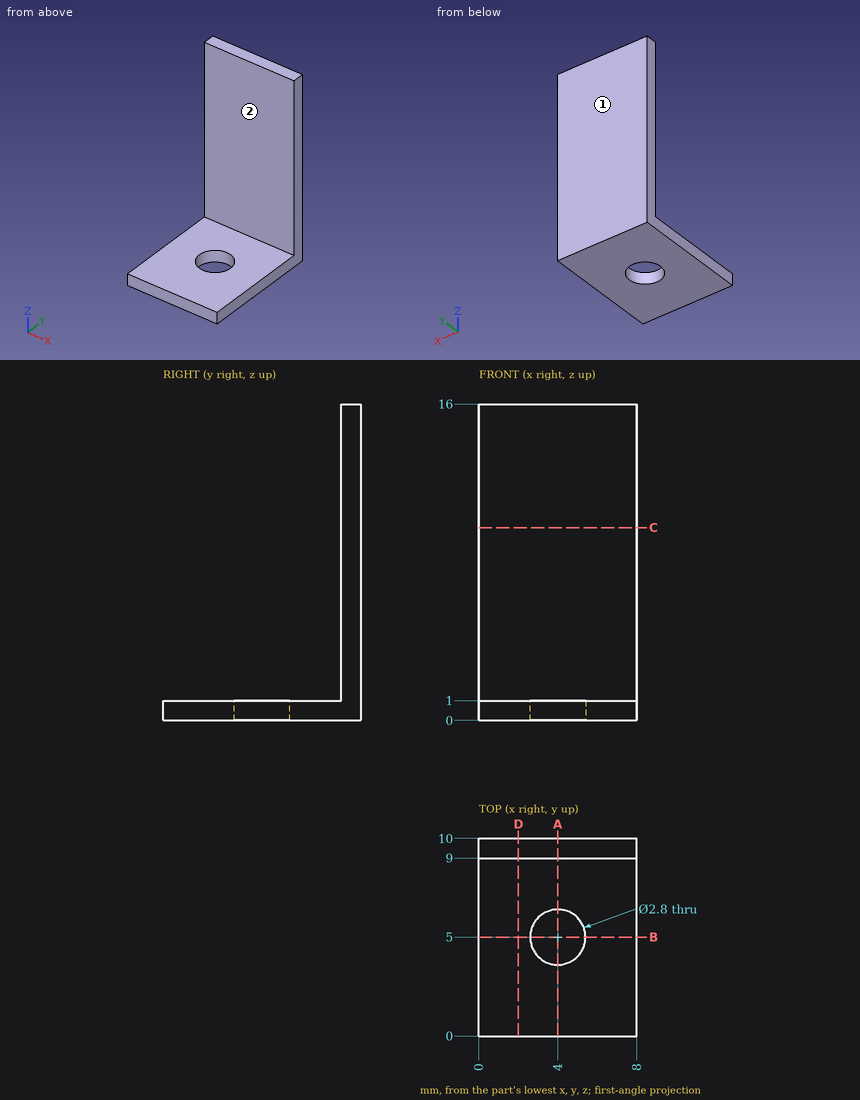
Source: three-view drawing plus pictorial views. Frame: mm from the lowest corner of the part. A direction names the side the tool comes from. Round coordinates to 2 decimals unless told otherwise and drop trailing zeros. Loops run counter-clockwise (first coordinate to the right, second up) from the corner with the lowest first, then second, coordinate; pieces in that order, holes last.
Q1. Section D-D, the plane x = 2. Return loops of the section in (y, z), plus the area to 3 significant figures.
Q2. Ray query, line 1 (Y direction, x = 4, z = 0.3); line 2 (Z direction, x = 6.5, y = 3); line 3 (Y direction, x = 1, z = 14.5). Return the intervals inside material, ascending.
Q3. Section C-C, the plane z = 9.75. Return loops of the section in (x, y), plus the area to 3 significant figures.
Q4. Section A-A, the plane x = 4. Return loops of the section in (y, z), plus the area to 3 significant figures.
Q5. Section B-B, the plane y = 5. Return loops of the section in (x, z).
Q6. Access query for the marked faces 1 and 2. Directions: +Z, -Z, +X, -X, +Y, -Y. A direction counts if a zero-diameter tool reaches every point of the face in a straight line with its end or side. Return the directions, or none.
Q7. First-contact query: P1, Ø2.5, axis at x = 4, y = 5, coming from the +Z side; P2, Ø2.5, axis at x = 4.5, z = 9, coming from the -Y side; P3, Ø4, axis at x = 2.5, y = 2, coming from the +Z side. Flat tips, straight axial feed; report the tip coordinate or a pass-through.
Solutions:
1. outline: (0, 0) - (10, 0) - (10, 16) - (9, 16) - (9, 1) - (0, 1) - close
1. area: 25.0 mm2
2. line 1: y = 0 to 3.6, 6.4 to 10
2. line 2: z = 0 to 1
2. line 3: y = 9 to 10
3. outline: (0, 9) - (8, 9) - (8, 10) - (0, 10) - close
3. area: 8.00 mm2
4. outline: (0, 0) - (3.6, 0) - (3.6, 1) - (0, 1) - close; (6.4, 0) - (10, 0) - (10, 16) - (9, 16) - (9, 1) - (6.4, 1) - close
4. area: 22.2 mm2
5. outline: (0, 0) - (2.6, 0) - (2.6, 1) - (0, 1) - close; (5.4, 0) - (8, 0) - (8, 1) - (5.4, 1) - close
6. face 1: +Z, -Z, +X, -X, +Y
6. face 2: +Z, +X, -X, -Y
7. P1: passes through
7. P2: stops at y = 9
7. P3: stops at z = 1
